Part model, mm, in its own coordinate system. A direction names the side the tool comes from. Round coordinates to 2 decimals unless told otherwise and drop trailing zeros. Write each loop counter-clockwise with the first axis right and the second up, starting at its lowest first coordinate (ties: lowest second). Pieces come first, ordered by that corner, then holes. Notation, with made-up numbers: M 29,86.25 L 52,86.25 A20 ccw 52,100.25 Z; hole C 12.5,0.25 d6. An arc over 180 degrees is marked long. Use a Markdown table: item, result. Add a question column.
1) Slice it at B-B on y = 20. Write the cut outline in (x, z), plus the area to 3 significant figures.
2) Slice it at D-D on y = 1. Write the cut outline in (x, z).
3) Two-plate mould, pull along Y, no slides. Class faces 1 (the face through (-4.629, -19, -10)), 2 (the face through (6.421, -6.624, -12.325)), 3 (the face through (-13.552, -0.521, 2.465)): released by +Y, released by -Y, zero draft, split by the parting line, or undercut.
4) Slice it at A-A on z = -10. Give the number of separate pieces and of enclosed holes in the cut face, plus the area to 3 significant figures.
5) Wall check: probe 1 along X at (y, z) = (14, -2); probe 2 along Y at (x, z) = (-11, -4); probe 3 along Z at (x, y) = (-6.5, -6). Give the ranges that are in metal, low to high.
6) Drop flat-ended pins along their axis: P1, Ø14.5, axis at x = -16, z = -8.5, coming from the -Y side; P2, Ø10, axis at x = 14, z = -6, coming from the +Y side; P3, Ø7, axis at y = 12, z = -9.5, coming from the +X side. Give the stop position or say it passes through.
7) Which spindle directions (+Z, -Z, +X, -X, +Y, -Y) get a long thin tool onto all of the face, cutting with end or side? Do faces 4 (the face through (5.049, -5.167, -12.325)), 5 (the face through (-15, -5.643, -10)), 6 (the face through (4.51, -27.26, 1.55)), 7 (the face through (6.6, 5.5, 0)), 8 (the face through (-19.59, 3.52, 1.55)). Say none if no direction does.
```python
from build123d import *

# Parameters (mm, degrees)
F1_DEPTH = 25
F2_W     = 6.15
F2_H     = 2
F2_W_2   = 2
F2_H_2   = 6.15
F3_DEPTH = 25
F5_DEPTH = 5
F6_R     = 0.75
F7_DEPTH = 5
F8_DEPTH = 5
F9_SIZE  = 7
F10_SIZE = 4.99999
F11_SIZE = 1


# Not quite as in the source:
# - a fillet or chamfer is up to 0.001 mm smaller than in the source, because OpenCascade refuses the exact size


with BuildPart() as f1:
    # F0 (on Top) → F1 (new body)
    with BuildSketch(Plane.XY):
        with BuildLine():
            Line((5.5211611295, 29.3387952344), (-4.6288388705, 29.3387952344))
            Line((-4.6288388705, 29.3387952344), (-4.6288388705, 5.9433882713))
            ThreePointArc((-4.6288388705, 5.9433882713), (-5.4099272548, 5.2703597245), (-6.1025520558, 4.5065944634))
            Line((-6.1025520558, 4.5065944634), (-23.141437278, 4.5065944634))
            Line((-23.141437278, 4.5065944634), (-23.141437278, -5.6434055366))
            Line((-23.141437278, -5.6434055366), (-6.3576590277, -5.6434055366))
            ThreePointArc((-6.3576590277, -5.6434055366), (-5.5589979581, -6.5937343191), (-4.6288388705, -7.4157978024))
            Line((-4.6288388705, -7.4157978024), (-4.6288388705, -30.8112047656))
            Line((-4.6288388705, -30.8112047656), (5.5211611295, -30.8112047656))
            Line((5.5211611295, -30.8112047656), (5.5211611295, -7.4157978024))
            ThreePointArc((5.5211611295, -7.4157978024), (6.4513202171, -6.5937343191), (7.2499812866, -5.6434055366))
            Line((7.2499812866, -5.6434055366), (23.7822366705, -5.6434055366))
            Line((23.7822366705, -5.6434055366), (23.7822366705, 4.5065944634))
            Line((23.7822366705, 4.5065944634), (6.9948743147, 4.5065944634))
            ThreePointArc((6.9948743147, 4.5065944634), (6.3022495138, 5.2703597245), (5.5211611295, 5.9433882713))
            Line((5.5211611295, 5.9433882713), (5.5211611295, 29.3387952344))
        make_face()
        with BuildLine():
            Line((-2.6288388705, 4.8639394003), (-2.6288388705, 27.3387952344))
            Line((-2.6288388705, 27.3387952344), (3.5211611295, 27.3387952344))
            Line((3.5211611295, 27.3387952344), (3.5211611295, 4.8639394003))
            ThreePointArc((3.5211611295, 4.8639394003), (4.8949803528, 3.8491247969), (5.9508403063, 2.5065944634))
            Line((5.9508403063, 2.5065944634), (21.7822366705, 2.5065944634))
            Line((21.7822366705, 2.5065944634), (21.7822366705, -3.6434055366))
            Line((21.7822366705, -3.6434055366), (6.1352228584, -3.6434055366))
            ThreePointArc((6.1352228584, -3.6434055366), (5.0303928567, -5.1861552316), (3.5211611295, -6.3363489315))
            Line((3.5211611295, -6.3363489315), (3.5211611295, -28.8112047656))
            Line((3.5211611295, -28.8112047656), (-2.6288388705, -28.8112047656))
            Line((-2.6288388705, -28.8112047656), (-2.6288388705, -6.3363489315))
            ThreePointArc((-2.6288388705, -6.3363489315), (-4.1380705978, -5.1861552316), (-5.2429005995, -3.6434055366))
            Line((-5.2429005995, -3.6434055366), (-21.141437278, -3.6434055366))
            Line((-21.141437278, -3.6434055366), (-21.141437278, 2.5065944634))
            Line((-21.141437278, 2.5065944634), (-5.0585180473, 2.5065944634))
            ThreePointArc((-5.0585180473, 2.5065944634), (-4.0026580939, 3.8491247969), (-2.6288388705, 4.8639394003))
        make_face(mode=Mode.SUBTRACT)
    extrude(amount=-F1_DEPTH)

    # F2 (on face) → F3 (cut, through all)
    with BuildSketch(Plane.XY):
        with Locations((0.4461611295, 28.3387952344)):
            Rectangle(F2_W, F2_H)
        with Locations((-22.141437278, -0.5684055366)):
            Rectangle(F2_W_2, F2_H_2)
        with Locations((22.7822366705, -0.5684055366)):
            Rectangle(F2_W_2, F2_H_2)
        with Locations((0.4461611295, -29.8112047656)):
            Rectangle(F2_W, F2_H)
    extrude(amount=-F3_DEPTH, mode=Mode.SUBTRACT)

    # F4 (on Top) → F5 (join)
    with BuildSketch(Plane.XY):
        with BuildLine():
            Line((3.5211611295, 4.8639394003), (3.5211611295, 12.9219201057))
            ThreePointArc((3.5211611295, 12.9219201057), (0.4461611295, 13.2637952344), (-2.6288388705, 12.9219201057))
            Line((-2.6288388705, 12.9219201057), (-2.6288388705, 4.8639394003))
            ThreePointArc((-2.6288388705, 4.8639394003), (-4.0026580939, 3.8491247969), (-5.0585180473, 2.5065944634))
            Line((-5.0585180473, 2.5065944634), (-13.1730992455, 2.5065944634))
            ThreePointArc((-13.1730992455, 2.5065944634), (-13.5527822586, -0.5642047132), (-13.2486621142, -3.6434055366))
            Line((-13.2486621142, -3.6434055366), (-5.2429005995, -3.6434055366))
            ThreePointArc((-5.2429005995, -3.6434055366), (-4.1380705978, -5.1861552316), (-2.6288388705, -6.3363489315))
            Line((-2.6288388705, -6.3363489315), (-2.6288388705, -14.3943296369))
            ThreePointArc((-2.6288388705, -14.3943296369), (0.4461611295, -14.7362047656), (3.5211611295, -14.3943296369))
            Line((3.5211611295, -14.3943296369), (3.5211611295, -6.3363489315))
            ThreePointArc((3.5211611295, -6.3363489315), (5.0303928567, -5.1861552316), (6.1352228584, -3.6434055366))
            Line((6.1352228584, -3.6434055366), (14.1409843732, -3.6434055366))
            ThreePointArc((14.1409843732, -3.6434055366), (14.3696579139, -2.1977920171), (14.4461611295, -0.7362047656))
            ThreePointArc((14.4461611295, -0.7362047656), (14.350650427, 0.8963323321), (14.0654215044, 2.5065944634))
            Line((14.0654215044, 2.5065944634), (5.9508403063, 2.5065944634))
            ThreePointArc((5.9508403063, 2.5065944634), (4.8949803528, 3.8491247969), (3.5211611295, 4.8639394003))
        make_face()
        with BuildLine():
            ThreePointArc((13.5579642318, -5.6434055366), (13.8867267431, -4.6542649982), (14.1409843732, -3.6434055366))
            Line((14.1409843732, -3.6434055366), (6.1352228584, -3.6434055366))
            ThreePointArc((6.1352228584, -3.6434055366), (5.0303928567, -5.1861552316), (3.5211611295, -6.3363489315))
            Line((3.5211611295, -6.3363489315), (3.5211611295, -14.3943296369))
            ThreePointArc((3.5211611295, -14.3943296369), (4.5325724418, -14.1265461573), (5.5211611295, -13.783977564))
            Line((5.5211611295, -13.783977564), (5.5211611295, -7.4157978024))
            ThreePointArc((5.5211611295, -7.4157978024), (6.4513202171, -6.5937343191), (7.2499812866, -5.6434055366))
            Line((7.2499812866, -5.6434055366), (13.5579642318, -5.6434055366))
        make_face()
        with BuildLine():
            Line((-4.6288388705, 5.9433882713), (-4.6288388705, 12.3115680329))
            ThreePointArc((-4.6288388705, 12.3115680329), (-9.3893111671, 9.2269014119), (-12.5350967543, 4.5065944634))
            Line((-12.5350967543, 4.5065944634), (-6.1025520558, 4.5065944634))
            ThreePointArc((-6.1025520558, 4.5065944634), (-5.4099272548, 5.2703597245), (-4.6288388705, 5.9433882713))
        make_face()
        with BuildLine():
            Line((-2.6288388705, 4.8639394003), (-2.6288388705, 12.9219201057))
            ThreePointArc((-2.6288388705, 12.9219201057), (-3.6402501828, 12.6541366261), (-4.6288388705, 12.3115680329))
            Line((-4.6288388705, 12.3115680329), (-4.6288388705, 5.9433882713))
            ThreePointArc((-4.6288388705, 5.9433882713), (-5.4099272548, 5.2703597245), (-6.1025520558, 4.5065944634))
            Line((-6.1025520558, 4.5065944634), (-12.5350967543, 4.5065944634))
            ThreePointArc((-12.5350967543, 4.5065944634), (-12.8916382733, 3.5185698574), (-13.1730992455, 2.5065944634))
            Line((-13.1730992455, 2.5065944634), (-5.0585180473, 2.5065944634))
            ThreePointArc((-5.0585180473, 2.5065944634), (-4.0026580939, 3.8491247969), (-2.6288388705, 4.8639394003))
        make_face()
        with BuildLine():
            ThreePointArc((13.4274190132, 4.5065944634), (10.281633426, 9.2269014119), (5.5211611295, 12.3115680329))
            Line((5.5211611295, 12.3115680329), (5.5211611295, 5.9433882713))
            ThreePointArc((5.5211611295, 5.9433882713), (6.3022495138, 5.2703597245), (6.9948743147, 4.5065944634))
            Line((6.9948743147, 4.5065944634), (13.4274190132, 4.5065944634))
        make_face()
        with BuildLine():
            Line((5.5211611295, 5.9433882713), (5.5211611295, 12.3115680329))
            ThreePointArc((5.5211611295, 12.3115680329), (4.5325724418, 12.6541366261), (3.5211611295, 12.9219201057))
            Line((3.5211611295, 12.9219201057), (3.5211611295, 4.8639394003))
            ThreePointArc((3.5211611295, 4.8639394003), (4.8949803528, 3.8491247969), (5.9508403063, 2.5065944634))
            Line((5.9508403063, 2.5065944634), (14.0654215044, 2.5065944634))
            ThreePointArc((14.0654215044, 2.5065944634), (13.7839605322, 3.5185698574), (13.4274190132, 4.5065944634))
            Line((13.4274190132, 4.5065944634), (6.9948743147, 4.5065944634))
            ThreePointArc((6.9948743147, 4.5065944634), (6.3022495138, 5.2703597245), (5.5211611295, 5.9433882713))
        make_face()
        with BuildLine():
            ThreePointArc((5.5211611295, -13.783977564), (10.4089508996, -10.5719975652), (13.5579642318, -5.6434055366))
            Line((13.5579642318, -5.6434055366), (7.2499812866, -5.6434055366))
            ThreePointArc((7.2499812866, -5.6434055366), (6.4513202171, -6.5937343191), (5.5211611295, -7.4157978024))
            Line((5.5211611295, -7.4157978024), (5.5211611295, -13.783977564))
        make_face()
        with BuildLine():
            Line((-6.3576590277, -5.6434055366), (-12.6656419728, -5.6434055366))
            ThreePointArc((-12.6656419728, -5.6434055366), (-9.5166286406, -10.5719975652), (-4.6288388705, -13.783977564))
            Line((-4.6288388705, -13.783977564), (-4.6288388705, -7.4157978024))
            ThreePointArc((-4.6288388705, -7.4157978024), (-5.5589979581, -6.5937343191), (-6.3576590277, -5.6434055366))
        make_face()
        with BuildLine():
            Line((-5.2429005995, -3.6434055366), (-13.2486621142, -3.6434055366))
            ThreePointArc((-13.2486621142, -3.6434055366), (-12.9944044841, -4.6542649982), (-12.6656419728, -5.6434055366))
            Line((-12.6656419728, -5.6434055366), (-6.3576590277, -5.6434055366))
            ThreePointArc((-6.3576590277, -5.6434055366), (-5.5589979581, -6.5937343191), (-4.6288388705, -7.4157978024))
            Line((-4.6288388705, -7.4157978024), (-4.6288388705, -13.783977564))
            ThreePointArc((-4.6288388705, -13.783977564), (-3.6402501828, -14.1265461573), (-2.6288388705, -14.3943296369))
            Line((-2.6288388705, -14.3943296369), (-2.6288388705, -6.3363489315))
            ThreePointArc((-2.6288388705, -6.3363489315), (-4.1380705978, -5.1861552316), (-5.2429005995, -3.6434055366))
        make_face()
    extrude(amount=F5_DEPTH)

    # F6 (on face) → F7 (cut, through all)
    with BuildSketch(Plane.XY.offset(5)):
        with Locations((0.4461611295, 10.2637952344)):
            Circle(F6_R)
        with Locations((0.4461611295, -11.7362047656)):
            Circle(F6_R)
    extrude(amount=-F7_DEPTH, mode=Mode.SUBTRACT)

    # F8 (add): faces of the model
    f8_faces = [f1.faces().sort_by_distance(p)[0] for p in [
        (-3.6349246548, 20.9904665399, 0),
        (4.5272469138, 20.9904665399, 0),
        (18.7764211463, 3.5172058862, 0),
        (18.8278982695, -4.6532031137, 0),
        (-18.0099019482, 3.5169457421, 0),
        (-18.0613729447, -4.6529604993, 0),
        (-3.6349246548, -22.4628760711, 0),
        (4.5272469138, -22.4628760711, 0),
    ]]
    extrude(f8_faces, amount=F8_DEPTH)

    # F9
    f9_edges = [f1.edges().sort_by_distance(p)[0] for p in [
        (-23.141437, 3.506594, 5),
        (-23.141437, -4.643406, 5),
        (-3.628839, -30.811205, 5),
        (4.521161, -30.811205, 5),
        (23.782237, -4.643406, 5),
        (23.782237, 3.506594, 5),
        (-3.628839, 29.338795, 5),
        (4.521161, 29.338795, 5),
    ]]
    chamfer(f9_edges, length=F9_SIZE)

    # F10 (size 5 in the source; OpenCascade refuses exactly that, so slightly less here)
    f10_edges = [f1.edges().sort_by_distance(p)[0] for p in [
        (10.281633, 9.226901, 0),
        (-9.389311, 9.226901, 0),
        (10.408951, -10.571998, 0),
        (-9.516629, -10.571998, 0),
    ]]
    chamfer(f10_edges, length=F10_SIZE)

    # F11
    f11_edges = [f1.edges().sort_by_distance(p)[0] for p in [
        (15.388555, 4.506594, -25),
        (5.521161, 17.641092, -25),
        (-4.628839, 17.641092, -25),
        (-14.621995, 4.506594, -25),
        (-14.749548, -5.643406, -25),
        (-4.628839, -19.113501, -25),
        (5.521161, -19.113501, -25),
        (15.516109, -5.643406, -25),
    ]]
    chamfer(f11_edges, length=F11_SIZE)


solid = f1.part
```
Entries:
| question | item | result |
|---|---|---|
| 1 | outline | M -4.63,-24 L -3.63,-25 L -2.63,-25 L -2.63,5 L -4.63,5 Z; M 3.52,-25 L 4.52,-25 L 5.52,-24 L 5.52,5 L 3.52,5 Z |
| 1 | area | 119 mm^2 |
| 2 | outline | M -13.45,0 L 14.34,0 L 14.34,5 L -13.45,5 Z |
| 3 | face 1 | zero draft |
| 3 | face 2 | released by -Y |
| 3 | face 3 | undercut |
| 4 | separate pieces | 4 |
| 4 | enclosed holes | 0 |
| 4 | area | 354 mm^2 |
| 5 | probe 1 | x = -4.63 to -2.63, 3.52 to 5.52 |
| 5 | probe 2 | y = -5.64 to -3.64, 2.51 to 4.51 |
| 5 | probe 3 | z = 0 to 5 |
| 6 | P1 | stops at y = -5.64 |
| 6 | P2 | stops at y = 4.51 |
| 6 | P3 | stops at x = 5.52 |
| 7 | face 4 | -Z |
| 7 | face 5 | -Z, -X, -Y |
| 7 | face 6 | +Z, +X, -X, -Y |
| 7 | face 7 | -Z, +X, +Y |
| 7 | face 8 | +Z, -X, +Y, -Y |
